Design review of the part shown in the three views and the two pictorial views. Dimensions are in mm from the part's minimum x, y and z. Coordinates: 2 decimals unless noted, no trailing zeros. Write each loop counter-clockwise with the first axis right and the second up, starting at its lowest first coordinate (ties: lowest second). Pieces come first, ordered by that corner, then holes. Notation, with made-up numbers: (57.25, -15.75) -> (80.25, -15.75) arc R18 ccw to (80.25, 17.25) -> close; hole circle Ø1 at (-34.5, 21.25). An arc over 180 degrees is marked (long way). Write each question's results on one line, items separated by ' | '.
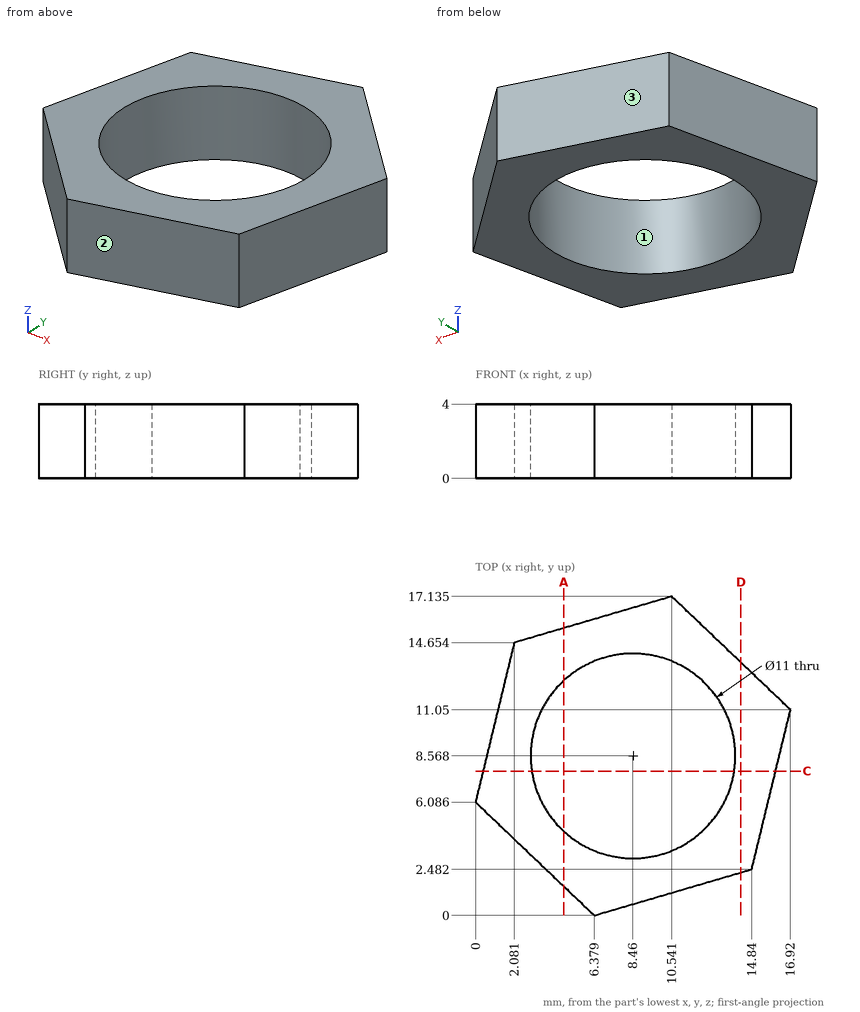
Q1. Add section D-D (x = 14.25). Write out the cut boundary in (y, z).
Solution:
outline: (2.31, 0) -> (13.6, 0) -> (13.6, 4) -> (2.31, 4) -> close
Q2. Clearance check with flat-ended pins moving along their axes: P1, Ø1, axis at y = 11, z = 2, coming from the +X side; P2, Ø6, axis at x = 8.5, y = 6.5, coming from the -Z side; P3, Ø2, axis at y = 2, z = 1, coming from the -X side (1 decimal). State where each tip first meets the part, or that it passes through.
Solution:
P1: x = 16.92 | P2: through | P3: x = 3.2
Q3. Add section C-C (y = 7.75). Write out the cut boundary in (x, z) (1 decimal).
Solution:
outline: (0.4, 0) -> (3, 0) -> (3, 4) -> (0.4, 4) -> close; (13.9, 0) -> (16.1, 0) -> (16.1, 4) -> (13.9, 4) -> close
Q4. Add section A-A (x = 4.75). Write out the cut boundary in (y, z) (1 decimal).
Solution:
outline: (1.6, 0) -> (4.5, 0) -> (4.5, 4) -> (1.6, 4) -> close; (12.6, 0) -> (15.4, 0) -> (15.4, 4) -> (12.6, 4) -> close
Q5. For line 1 (Y direction, x = 10, z = 3.3); line 2 (X direction, y = 7.25, z = 2.9); line 3 (X direction, y = 12, z = 0.65) (1 decimal), list the stretches that pass through material, from the lowest coordinate up. Write a range as from..to.
Solution:
line 1: 1.06..3.29, 13.85..16.98 | line 2: 0.28..3.12, 13.8..16 | line 3: 1.4..4.2, 12.8..15.9
Q6. Draft analysis for pull direction Y (two halves, no side actions). For the marked faces 1, 2 and 3, state which applies: pulls with the +Y half, pulls with the -Y half, needs draft (parallel to the pull), parting line crosses it, or undercut.
Solution:
face 1: undercut | face 2: pulls with the -Y half | face 3: pulls with the +Y half
